Can you work these out from the model? Positions are in its coordinate system, mm. Face numbers are marked on the shaded views. A direction names the side the tool comes from. Round coordinates to 2 decimals unless told otherwise and drop trailing zeros. Order: outer loops, then holes, each group sorted by start corner. A loop starts at its lowest first (then second) coordinate and runs counter-clockwise, first axis right, second up.
Q1. If we section it at A-A (y = 7): Please give me the cut outline in (x, z).
Q2. If we section it at D-D (x = -1.75): Please give me the cut outline in (y, z), plus the area to 3 significant figures.
Q3. For the marked faces 4, 5 and 6, which set-ups out of +Z, -Z, +X, -X, +Y, -Y let a thin tool reach every point of the face, with its end or its side?
Q4. We'd pull the mould along X, two halves only. Please class the marked faces 1, 2 and 3: pulls with the +X half, pulls with the -X half, needs draft (parallel to the pull), parting line crosses it, or undercut.
Q5. If we section it at C-C (z = 11): Please give me the cut outline in (x, y), plus the area to 3 significant figures.
Q6. Will these pins go through, and if not, where does the flat tip stop? P1, Ø3, axis at x = -17, z = 13, coming from the +Y side; P2, Ø4, axis at x = -3.5, y = 18.5, coming from the -Z side; P3, Ø3, axis at x = -8.5, y = 20.5, coming from the -Z side.
Q7. If I drill on line 1 (Y direction, x = -18.5, z = 28); line 2 (Y direction, x = -18, z = 16.5); line 3 (X direction, y = 10.5, z = 7), over which ranges is the centre line in solid material (lowest first)?
Q8. If we section it at B-B (y = 18.75): Please give me the cut outline in (x, z), plus the area to 3 significant figures.
Autodesk Inventor part; units mm, degrees
ref_plane "YZ Plane" through (0, 0, 0) normal (1, 0, 0) x (0, 1, 0)
ref_plane "XZ Plane" through (0, 0, 0) normal (0, 1, 0) x (-1, 0, 0)
ref_plane "XY Plane" through (0, 0, 0) normal (0, 0, 1) x (1, 0, 0)
sketch "Sketch1" plane through (0, 0, 0) normal (0, 1, 0) x (-1, 0, 0)
  line L0 (0, 0) -> (22.86, 0)
  line L1 (22.86, 0) -> (22.86, 35.56)
  line L2 (22.86, 35.56) -> (0, 35.56)
  line L3 (0, 35.56) -> (0, 0)
  dimension "d0" = 22.86
  dimension "d1" = 35.56
extrude "Extrusion1" add sketch "Sketch1" along normal blind 15.24
sketch "Sketch2" plane through (-22.86, 0, 35.56) normal (0, 0, 1) x (1, 0, 0)
  line L0 (2.54, 2.54) -> (20.32, 2.54)
  line L1 (20.32, 2.54) -> (20.32, 12.7)
  line L2 (20.32, 12.7) -> (2.54, 12.7)
  line L3 (2.54, 12.7) -> (2.54, 2.54)
  point P0 (0, 0)
  dimension "d6" = 17.78
  dimension "d7" = 10.16
extrude "Extrusion2" cut sketch "Sketch2" against normal blind 33.02
sketch "Sketch5" plane through (0, 15.24, 0) normal (0, 1, 0) x (1, 0, 0)
  line L0 (-22.86, -35.56) -> (0, -35.56)
  line L1 (0, -35.56) -> (0, 0)
  line L2 (-22.86, -35.56) -> (0, -35.56)
  line L3 (0, -35.56) -> (0, -17.78)
  line L4 (0, -17.78) -> (-22.86, -17.78)
  line L5 (-22.86, -17.78) -> (-22.86, -35.56)
extrude "Extrusion5" add sketch "Sketch5" along normal blind 10.16
sketch "Sketch10" plane through (-22.86, 0, 35.56) normal (0, 0, 1) x (1, 0, 0)
  line L0 (2.54, 15.24) -> (20.32, 15.24)
  line L1 (20.32, 15.24) -> (20.32, 22.86)
  line L2 (20.32, 22.86) -> (2.54, 22.86)
  line L3 (2.54, 22.86) -> (2.54, 15.24)
  line L4 (2.54, 12.7) -> (20.32, 12.7)
  line L5 (22.86, 0) -> (22.86, 25.4)
  dimension "d27" = 17.78
  dimension "d28" = 7.62
  dimension "d29" = 2.54
  dimension "d30" = 2.54
sketch "Sketch11" plane through (0, 15.24, 17.78) normal (0, 0, -1) x (-1, 0, 0)
  line L0 (17.78, 7.62) -> (5.08, 7.62)
  line L1 (5.08, 7.62) -> (5.08, 0)
  line L2 (5.08, 0) -> (17.78, 0)
  line L3 (17.78, 0) -> (17.78, 7.62)
  line L4 (0, 10.16) -> (22.86, 10.16)
  line L5 (22.86, 0) -> (22.86, 10.16)
  point P0 (0, -15.24)
  dimension "d31" = 2.54
  dimension "d33" = 5.08
  dimension "d35" = 12.7
  dimension "d36" = 7.62
loft "Loft1" cut profiles "Sketch11", "Sketch10"
sketch "Sketch12" plane through (0, 0, 0) normal (0, 0, -1) x (-1, 0, 0)
  line L0 (22.86, 0) -> (0, 0)
  line L1 (0, 0) -> (11.43, 0)
  line L2 (11.43, 0) -> (11.43, 7.62)
  circle A0 centre (11.43, 7.62) radius 2.54
  dimension "d41" = 11.43
  dimension "d42" = 7.62
  dimension "d43" = 5.08
extrude "Extrusion8" cut sketch "Sketch12" against normal blind 25.4
sketch "Sketch13" plane through (0, 0, 0) normal (0, -1, 0) x (1, 0, 0)
  line L0 (0, 0) -> (-8.89, 0)
  line L1 (0, 0) -> (-22.86, 0)
  line L2 (-22.86, 0) -> (-13.97, 0)
  line L3 (-20.32, 35.56) -> (-2.54, 35.56)
  line L4 (-13.97, 0) -> (-8.89, 0)
  line L5 (-8.89, 0) -> (-8.89, 35.56)
  line L6 (-8.89, 35.56) -> (-13.97, 35.56)
  line L7 (-13.97, 35.56) -> (-13.97, 0)
  dimension "d46" = 8.89
  dimension "d47" = 8.89
extrude "Extrusion9" cut sketch "Sketch13" against normal blind 7.62
properties part number "big usb cover"
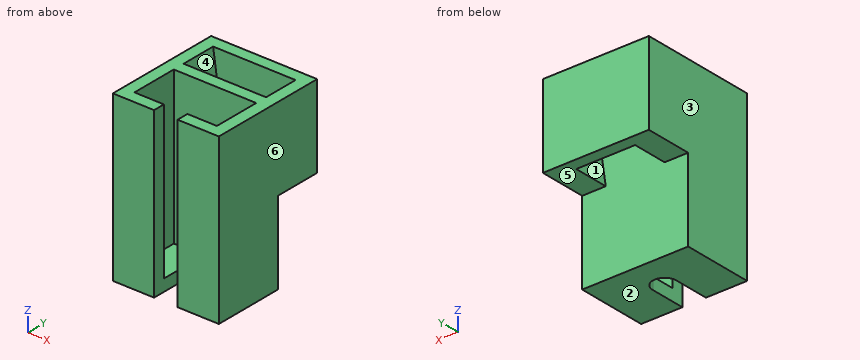
Solution:
1. outline: (-22.86, 0) - (-13.97, 0) - (-13.97, 2.54) - (-20.32, 2.54) - (-20.32, 35.56) - (-22.86, 35.56) - close; (-8.89, 0) - (0, 0) - (0, 35.56) - (-2.54, 35.56) - (-2.54, 2.54) - (-8.89, 2.54) - close
2. outline: (0, 0) - (15.24, 0) - (15.24, 17.78) - (25.4, 17.78) - (25.4, 35.56) - (0, 35.56) - close
2. area: 723 mm2
3. face 4: +Z
3. face 5: -Z, +X, -X, +Y
3. face 6: +Z, -Z, +X, +Y, -Y
4. face 1: undercut
4. face 2: needs draft
4. face 3: pulls with the -X half
5. outline: (-22.86, 0) - (-13.97, 0) - (-13.97, 2.54) - (-20.32, 2.54) - (-20.32, 12.7) - (-2.54, 12.7) - (-2.54, 2.54) - (-8.89, 2.54) - (-8.89, 0) - (0, 0) - (0, 15.24) - (-22.86, 15.24) - close
5. area: 155 mm2
6. P1: stops at y = 15.24
6. P2: stops at z = 17.78
6. P3: passes through
7. line 1: y = 0 to 2.54, 12.7 to 15.24, 22.86 to 25.4
7. line 2: y = 0 to 2.54, 12.7 to 15.24
7. line 3: x = -22.86 to -20.32, -2.54 to 0
8. outline: (-22.86, 17.78) - (-17.78, 17.78) - (-20.32, 35.56) - (-22.86, 35.56) - close; (-5.08, 17.78) - (0, 17.78) - (0, 35.56) - (-2.54, 35.56) - close
8. area: 135 mm2
